from build123d import *

# Parameters (mm, degrees)
SKETCH2_R                                       = 7.5
BOSS_EXTRUDE1_DEPTH                             = 10
CSK_FOR_M4_FLAT_HEAD_MACHINE_SCREW1_D           = 4.3
CSK_FOR_M4_FLAT_HEAD_MACHINE_SCREW1_CSINK_D     = 11.4
CSK_FOR_M4_FLAT_HEAD_MACHINE_SCREW1_CSINK_ANGLE = 90
FILLET1_R                                       = 20
V_GROOVE_CUTOUT_DEPTH                           = 3.6
STANDARD_TAPERED_INSERT_CUTOUT_DEPTH            = 55.436206513
STANDARD_TAPERED_INSERT_CUTOUT_DEPTH_BACK       = 55.436206513
SKETCH13_R                                      = 2.25
TAPER_FOR_INSERTS_SIZE                          = 0.4
TAPER_FOR_INSERTS_SIZE2                         = 1.098990968
MOVE_FACE1_BY                                   = 0.5
MOVE_FACE1_2_BY                                 = 0.5
MOVE_FACE1_3_BY                                 = 0.5
MOVE_FACE1_4_BY                                 = 0.5
MOVE_FACE1_5_BY                                 = 0.5
MOVE_FACE1_6_BY                                 = 0.5
CIRPATTERN2_COUNT                               = 3
SKETCH47_R                                      = 1.6
CUT_EXTRUDE1_DEPTH                              = 55.436206513
CSK_FOR_M4_FLAT_HEAD_MACHINE_SCREW2_D           = 4.5
CSK_FOR_M4_FLAT_HEAD_MACHINE_SCREW2_DEPTH       = 10.1
CSK_FOR_M4_FLAT_HEAD_MACHINE_SCREW2_CSINK_D     = 9.4
CSK_FOR_M4_FLAT_HEAD_MACHINE_SCREW2_CSINK_ANGLE = 90
CSK_FOR_M4_FLAT_HEAD_MACHINE_SCREW2_TIP         = 1.351936393
FILLET2_R                                       = 3


with BuildPart() as part:
    # Sketch2 → Boss-Extrude1 (new body)
    with BuildSketch(Plane.XY):
        Polygon((-24.25, 40), (24.25, 40), (24.25, -5.917840259), (35.54293994, -12.437822174), (29.54293994, -22.830127019), (-29.54293994, -22.830127019), (-35.54293994, -12.437822174), (-24.25, -5.917840259), align=None)
        Circle(SKETCH2_R, mode=Mode.SUBTRACT)
    extrude(amount=BOSS_EXTRUDE1_DEPTH)

    # CSK for M4 Flat Head Machine Screw1 (through all)
    with Locations(Plane.XY.offset(10)):
        with Locations((-25.980762114, -15), (0, 30), (25.980762114, -15)):
            CounterSinkHole(CSK_FOR_M4_FLAT_HEAD_MACHINE_SCREW1_D / 2, CSK_FOR_M4_FLAT_HEAD_MACHINE_SCREW1_CSINK_D / 2, counter_sink_angle=CSK_FOR_M4_FLAT_HEAD_MACHINE_SCREW1_CSINK_ANGLE)

    # Fillet1
    fillet1_edges = [part.edges().sort_by_distance(p)[0] for p in [
        (24.25, -5.917840259, 5),
        (-24.25, -5.917840259, 5),
    ]]
    fillet(fillet1_edges, radius=FILLET1_R)

    # Sketch44 → v-groove cutout (cut)
    with BuildSketch(Plane(origin=(0, 0, 0), x_dir=(-1, 0, 0), z_dir=(0, 0, -1))):
        with BuildLine():
            Line((10.392304845, 10), (-10.392304845, 10))
            ThreePointArc((-10.392304845, 10), (-13.856406461, 8), (-13.856406461, 4))
            Line((-13.856406461, 4), (-3.464101615, -14))
            ThreePointArc((-3.464101615, -14), (0, -16), (3.464101615, -14))
            Line((3.464101615, -14), (13.856406461, 4))
            ThreePointArc((13.856406461, 4), (13.856406461, 8), (10.392304845, 10))
        make_face()
    extrude(amount=-V_GROOVE_CUTOUT_DEPTH, mode=Mode.SUBTRACT)

    # Sketch13 → standard tapered insert cutout (cut, two sides: drawn at the far end of the back side and taken through both)
    with BuildSketch(Plane(origin=(0, 0, 0), x_dir=(-1, 0, 0), z_dir=(0, 0, -1)).offset(-STANDARD_TAPERED_INSERT_CUTOUT_DEPTH_BACK)):
        with Locations((-10.392304845, 6)):
            Circle(SKETCH13_R)
        with Locations((10.392304845, 6)):
            Circle(SKETCH13_R)
        with Locations((0, -12)):
            Circle(SKETCH13_R)
    extrude(amount=STANDARD_TAPERED_INSERT_CUTOUT_DEPTH + STANDARD_TAPERED_INSERT_CUTOUT_DEPTH_BACK, mode=Mode.SUBTRACT)

    # taper for inserts
    taper_for_inserts_edges = [part.edges().sort_by_distance(p)[0] for p in [
        (12.642304845, 6, 10),
        (-8.142304845, 6, 10),
        (2.25, -12, 10),
    ]]
    taper_for_inserts_side = [part.faces().sort_by_distance(p)[0] for p in [
        (0, 7.937962268, 10),
    ]]
    chamfer(taper_for_inserts_edges, length=TAPER_FOR_INSERTS_SIZE, length2=TAPER_FOR_INSERTS_SIZE2, reference=taper_for_inserts_side[0])

    # Move Face1: a face moved inward by 0.5
    extrude(part.faces().sort_by_distance((-8.660254038, -5, 1.8))[0], amount=MOVE_FACE1_BY, dir=(-0.866025404, -0.5, 0), mode=Mode.SUBTRACT)

    # Move Face1 2: a curved face moved inward by 0.5
    add(Solid.thicken(part.faces().sort_by_distance((0, -16, 1.8))[0], -MOVE_FACE1_2_BY), mode=Mode.SUBTRACT)

    # Move Face1 3: a face moved inward by 0.5
    extrude(part.faces().sort_by_distance((8.660254038, -5, 1.8))[0], amount=MOVE_FACE1_3_BY, dir=(0.866025404, -0.5, 0), mode=Mode.SUBTRACT)

    # Move Face1 4: a curved face moved inward by 0.5
    add(Solid.thicken(part.faces().sort_by_distance((13.856406461, 8, 1.8))[0], -MOVE_FACE1_4_BY), mode=Mode.SUBTRACT)

    # Move Face1 5: a curved face moved inward by 0.5
    add(Solid.thicken(part.faces().sort_by_distance((-13.856406461, 8, 1.8))[0], -MOVE_FACE1_5_BY), mode=Mode.SUBTRACT)

    # Move Face1 6: a face moved inward by 0.5
    extrude(part.faces().sort_by_distance((0, 10, 1.8))[0], amount=MOVE_FACE1_6_BY, dir=(0, 1, 0), mode=Mode.SUBTRACT)

    # Sketch46 → tool ball cutout (revolve, cut)
    with BuildSketch(Plane(origin=(0, 30, 0), x_dir=(1, 0, 0), z_dir=(0, 1, 0))):
        with BuildLine():
            Line((0, 5.3), (0, -4.7))
            ThreePointArc((0, -4.7), (-5, 0.3), (0, 5.3))
        make_face()
    tool_ball_cutout = revolve(axis=Axis((0, 30, 0), (0, 0, -1)), mode=Mode.SUBTRACT)

    # CirPattern2: tool ball cutout ×3 about axis
    cirpattern2_axis = Axis((0, 0, 0), (0, 0, 1))
    for i in range(1, CIRPATTERN2_COUNT):
        add(tool_ball_cutout.rotate(cirpattern2_axis, i * 360 / CIRPATTERN2_COUNT), mode=Mode.SUBTRACT)

    # Sketch47 → Cut-Extrude1 (cut, through all)
    with BuildSketch(Plane(origin=(0, 0, 0), x_dir=(-1, 0, 0), z_dir=(0, 0, -1))):
        with Locations((-15.5, 18.269872981)):
            Circle(SKETCH47_R)
        with Locations((15.5, 18.269872981)):
            Circle(SKETCH47_R)
    extrude(amount=-CUT_EXTRUDE1_DEPTH, mode=Mode.SUBTRACT)

    # CSK for M4 Flat Head Machine Screw2
    with Locations(Plane(origin=(0, 0, 0), x_dir=(-1, 0, 0), z_dir=(0, 0, -1))):
        with Locations((-15.5, 29.134936491), (0, 18.269872981), (15.5, 29.134936491)):
            CounterSinkHole(CSK_FOR_M4_FLAT_HEAD_MACHINE_SCREW2_D / 2, CSK_FOR_M4_FLAT_HEAD_MACHINE_SCREW2_CSINK_D / 2, depth=CSK_FOR_M4_FLAT_HEAD_MACHINE_SCREW2_DEPTH, counter_sink_angle=CSK_FOR_M4_FLAT_HEAD_MACHINE_SCREW2_CSINK_ANGLE)
            with Locations((0, 0, -(CSK_FOR_M4_FLAT_HEAD_MACHINE_SCREW2_DEPTH + CSK_FOR_M4_FLAT_HEAD_MACHINE_SCREW2_TIP / 2))):  # 118° drill point
                Cone(0, CSK_FOR_M4_FLAT_HEAD_MACHINE_SCREW2_D / 2, CSK_FOR_M4_FLAT_HEAD_MACHINE_SCREW2_TIP, mode=Mode.SUBTRACT)

    # Fillet2
    fillet2_edges = [part.edges().sort_by_distance(p)[0] for p in [
        (24.25, 40, 5),
        (-24.25, 40, 5),
        (-29.54293994, -22.830127019, 5),
        (-35.54293994, -12.437822174, 5),
        (29.54293994, -22.830127019, 5),
        (35.54293994, -12.437822174, 5),
    ]]
    fillet(fillet2_edges, radius=FILLET2_R)


solid = part.part
For this review, take the finished solid that the model builds, in its own axes (mm). A direction names the side the tool comes from. Give positions to 0.01 mm unless a question says otherwise; leave off trailing zeros. Put each result on its own line as item: value. Start each with the question number.
(1) Wall thickness on L1, parallel to Y at x = 0, z = 5.2; L2, parallel to Y at x = -15.5, z = 4.75; L3, parallel to X at y = -15, z = 4.95: over which ranges is each line inside the solid? List them lowest first.
(2) The part is to be moulded in two halves that separate along X. For faces 3 (the cylindrical face through (-29.33, -22.417, 5.07)), 4 (the flat face through (0, 10.5, 2)), 5 (the flat face through (0, -22.83, 5)), 6 (the cylindrical face through (-0.3, 20.5, 6.3)), say which applies: +X half, -X half, draft (parallel to the pull), parting line (faces both ways), or undercut.
(3) Machinability: for faces 1 (the cylindrical face through (0.1, -16.5, 1.8)), 2 (the cylindrical face through (27.687, -16.308, 5.316)), which of the approach directions +Z, -Z, +X, -X, +Y, -Y give a long, thin tool a straight path to every point of the face, cutting with its end or side? Answer none if there is none.
(4) Add section A-A, the plane x = 0. Give the number of separate pieces and of enclosed holes in the cut face, then the cut area to 3 significant figures.
(5) For pin 1 (6 mm diameter, centred on x = 0, y = -12, fed in from -Z); pin 2 (3 mm diameter, centred on y = -11.5, z = 6, fed in from +X); pin 3 (7 mm diameter, centred on x = -25.98, y = -15, fed in from -Z), all flat-tipped, find the tip position at first contact; note any pin that passes through.
Result:
1. L1: y = -22.83 to -14.25, -9.75 to -7.5, 7.5 to 16.02, 20.52 to 27.85, 32.15 to 40
1. L2: y = -22.83 to 16.67, 19.87 to 26.88, 31.38 to 40
1. L3: x = -34.06 to -28.13, -23.83 to 23.83, 28.13 to 34.06
2. face 3: -X half
2. face 4: undercut
2. face 5: draft
2. face 6: undercut
3. face 1: -Z
3. face 2: +Z, -Z
4. separate pieces: 5
4. enclosed holes: 0
4. area: 283 mm^2
5. pin 1: stops at z = 3.6
5. pin 2: stops at x = 34.43
5. pin 3: stops at z = 3.27
